The listing builds one solid part. Answer for the finished solid, in the listing's coordinates (mm). A direction names the side the tool comes from. Round coordinates to 2 decimals unless told otherwise and drop trailing zeros. Order: outer loops, then holes, each group sorted by start corner. A loop starts at its lowest first (then second) coordinate and runs counter-clockwise, first axis right, second up. Notation, with made-up numbers: (-8, -2) - (43, -2) arc R23 ccw to (43, 28) - close; hole circle Ø4 at (82.5, 44). An arc over 180 degrees is marked (long way). One line per item, written item: value. Start each with the question number.
1. Section A-A, the plane x = -56 is taken. Give the vertices of the cut face in (y, z), then the cut area to 3 significant figures.
2. For a pull along X with two mould halves and no side action, classify faces 1 (the flat face through (-68.606, 3.986, 43.172)), 2 (the flat face through (-50.235, 1.479, 25.674)), 3 (the flat face through (-24, 1, 66.729)) as released by +X, released by -X, zero draft, split by the parting line, or undercut.
3. A tool of negligible diameter and unlimited length cuts with its end or side. For faces 4 (the conical face through (-9.466, 4.43, 62.722)), 5 (the flat face through (-45.45, 1.48, 60.39)), from which of +Z, -Z, +X, -X, +Y, -Y can it reach the whole face along a straight path? Write none if from no direction.
4. Section D-D, the plane x = -35 is taken. Give the vertices of the cut face in (y, z), then the cut area to 3 significant figures.
5. Section B-B, the plane x = -21.5 is taken. Give the vertices of the cut face in (y, z), then the cut area to 3 significant figures.
6. Straight lines are drawn through the part: line 1 (Z direction, x = -48, y = 1.3); line 2 (X direction, y = 3.6, z = 27); line 3 (Z direction, x = -28, y = 2.9). For each, find the intervals that lie inside material, in ascending order.
7. Section C-C, the plane z = 45 is taken. Count the separate pieces of the cut face and the enclosed holes in it, then the cut area to 3 significant figures.
8. Flat-ended cylindrical pins translate along their axes: P1, Ø4.5, axis at x = -14.09, z = 43.68, coming from the -Y side; P2, Ø8.5, axis at x = -17.59, z = 31.13, coming from the -Y side; P3, Ø5, axis at x = -47.84, z = 59.03, coming from the -Y side. Find the tip coordinate at first contact, or state that the pin passes through.
from build123d import *

# Parameters (mm, degrees)
SKETCH1_W           = 64
SKETCH1_H           = 47.5
SKETCH1_R           = 1.6
SKETCH1_R_2         = 3.75
BOSS_EXTRUDE1_DEPTH = 5
SKETCH2_R           = 1.6
CUT_EXTRUDE1_DEPTH  = 6
CUT_EXTRUDE2_DEPTH  = 3
FILLET1_R           = 10
FILLET2_R           = 10
CHAMFER1_SIZE       = 2
CHAMFER2_SIZE       = 1
SKETCH4_R           = 5.25
SKETCH4_R_2         = 7.5
CUT_EXTRUDE3_DEPTH  = 4


with BuildPart() as part:
    # Sketch1 → Boss-Extrude1 (new body)
    with BuildSketch(Plane(origin=(0, 0, 0), x_dir=(1, 0, 0), z_dir=(0, 1, 0))):
        with Locations((-37.591918828, -42.97941453)):
            Rectangle(SKETCH1_W, SKETCH1_H)
        with Locations((-39.091918828, -33.57941453)):
            Circle(SKETCH1_R, mode=Mode.SUBTRACT)
        with Locations((-56.591918828, -52.47941453)):
            Circle(SKETCH1_R, mode=Mode.SUBTRACT)
        with Locations((-28.091918828, -43.67941453)):
            Circle(SKETCH1_R_2, mode=Mode.SUBTRACT)
        with Locations((-14.091918828, -43.67941453)):
            Circle(SKETCH1_R_2, mode=Mode.SUBTRACT)
    extrude(amount=BOSS_EXTRUDE1_DEPTH)

    # Sketch2 → Cut-Extrude1 (cut, through all)
    with BuildSketch(Plane.XZ):
        with Locations((-47.841918828, 59.02941453)):
            Circle(SKETCH2_R)
        with Locations((-47.841918828, 27.02941453)):
            Circle(SKETCH2_R)
    extrude(amount=-CUT_EXTRUDE1_DEPTH, mode=Mode.SUBTRACT)

    # Sketch3 → Cut-Extrude2 (cut)
    with BuildSketch(Plane(origin=(0, 0, 0), x_dir=(-1, 0, 0), z_dir=(0, -1, 0))):
        Polygon((49.429632069, -56.27941453), (46.254205588, -56.27941453), (44.666492348, -59.02941453), (46.254205588, -61.77941453), (49.429632069, -61.77941453), (51.017345309, -59.02941453), align=None)
        Polygon((46.254205588, -29.77941453), (49.429632069, -29.77941453), (51.017345309, -27.02941453), (49.429632069, -24.27941453), (46.254205588, -24.27941453), (44.666492348, -27.02941453), align=None)
    extrude(amount=-CUT_EXTRUDE2_DEPTH, mode=Mode.SUBTRACT)

    # Fillet1
    fillet1_edges = [part.edges().sort_by_distance(p)[0] for p in [
        (-69.591918828, 2.5, 19.22941453),
        (-5.591918828, 2.5, 19.22941453),
    ]]
    fillet(fillet1_edges, radius=FILLET1_R)

    # Fillet2
    fillet2_edges = [part.edges().sort_by_distance(p)[0] for p in [
        (-5.591918828, 2.5, 66.72941453),
        (-69.591918828, 2.5, 66.72941453),
    ]]
    fillet(fillet2_edges, radius=FILLET2_R)

    # Chamfer1
    chamfer1_edges = [part.edges().sort_by_distance(p)[0] for p in [
        (-37.591918828, 5, 19.22941453),
        (-69.591918828, 5, 42.97941453),
        (-66.66298664, 5, 22.158346718),
        (-8.520851016, 5, 22.158346718),
        (-5.591918828, 5, 42.97941453),
        (-37.591918828, 5, 66.72941453),
        (-66.66298664, 5, 63.800482342),
        (-8.520851016, 5, 63.800482342),
    ]]
    chamfer(chamfer1_edges, length=CHAMFER1_SIZE)

    # Chamfer2
    chamfer2_edges = [part.edges().sort_by_distance(p)[0] for p in [
        (-17.841918828, 0, 43.67941453),
        (-31.841918828, 0, 43.67941453),
    ]]
    chamfer(chamfer2_edges, length=CHAMFER2_SIZE)

    # Sketch4 → Cut-Extrude3 (cut)
    with BuildSketch(Plane(origin=(0, 0, 0), x_dir=(1, 0, 0), z_dir=(0, 1, 0))):
        with Locations((-57.591918828, -31.12941453)):
            Circle(SKETCH4_R)
        with Locations((-17.591918828, -31.12941453)):
            Circle(SKETCH4_R)
        with Locations((-37.591918828, -71.32941453)):
            Circle(SKETCH4_R_2)
    extrude(amount=CUT_EXTRUDE3_DEPTH, mode=Mode.SUBTRACT)


solid = part.part
Answer list:
1. outline: (0, 19.23) - (3, 19.23) - (5, 21.23) - (5, 50.99) - (0, 50.99) - (0, 36.13) - (4, 36.13) - (4, 26.13) - (0, 26.13) - close; (0, 53.97) - (5, 53.97) - (5, 64.73) - (3, 66.73) - (0, 66.73) - close
1. area: 179 mm²
2. face 1: released by -X
2. face 2: undercut
2. face 3: zero draft
3. face 4: +Z, +X, +Y
3. face 5: -Y
4. outline: (0, 19.23) - (3, 19.23) - (5, 21.23) - (5, 64.73) - (4, 65.73) - (4, 64.29) - (0, 64.29) - close
4. area: 224 mm²
5. outline: (0, 19.23) - (3, 19.23) - (5, 21.23) - (5, 64.73) - (3, 66.73) - (0, 66.73) - (0, 34.64) - (4, 34.64) - (4, 27.62) - (0, 27.62) - close
5. area: 205 mm²
6. line 1: z = 19.23 to 24.28, 29.78 to 56.28, 61.78 to 66.73
6. line 2: x = -68.72 to -60.83, -54.35 to -49.44, -46.24 to -20.83, -14.35 to -6.46
6. line 3: z = 19.23 to 39.93, 47.43 to 66.73
7. separate pieces: 3
7. enclosed holes: 0
7. area: 244 mm²
8. P1: passes through
8. P2: stops at y = 4
8. P3: stops at y = 3
